Part model, mm, in its own coordinate system. Face numbers are marked on the shaded views. A direction names the side the tool comes from. Coordinates: 2 decimals unless noted, no trailing zeros. Order: outer loops, then holes, each group sorted by start corner. A loop starts at its lowest first (then second) coordinate and runs counter-clockwise, first axis right, second up. Notation, with made-up numbers: M 77,44.5 L 123,44.5 A33 ccw 123,74.5 Z; hole C -10,71.5 d6. An arc over 180 degrees is marked long. Answer in a Markdown table with one row per item. Add a question column.
from build123d import *

# Parameters (mm, degrees)
F0_W     = 6.2
F0_H     = 6.8
F1_DEPTH = 1.5
F2_R     = 1.8
F3_DEPTH = 0.5
F4_R     = 1.5
F5_DEPTH = 1
F6_SIZE  = 0.3


with BuildPart() as f1:
    # F0 (on Top) → F1 (new body)
    with BuildSketch(Plane.XY):
        Rectangle(F0_W, F0_H)
    extrude(amount=F1_DEPTH)

    # F2 (on face) → F3 (cut)
    with BuildSketch(Plane.XY.offset(1.5)):
        Circle(F2_R)
    extrude(amount=-F3_DEPTH, mode=Mode.SUBTRACT)

    # F4 (on face) → F5 (join)
    with BuildSketch(Plane.XY.offset(1)):
        Circle(F4_R)
    extrude(amount=F5_DEPTH)

    # F6
    f6_edges = [f1.edges().sort_by_distance(p)[0] for p in [
        (-3.1, -3.4, 0.75),
        (3.1, -3.4, 0.75),
        (3.1, 3.4, 0.75),
        (-3.1, 3.4, 0.75),
    ]]
    chamfer(f6_edges, length=F6_SIZE)


solid = f1.part
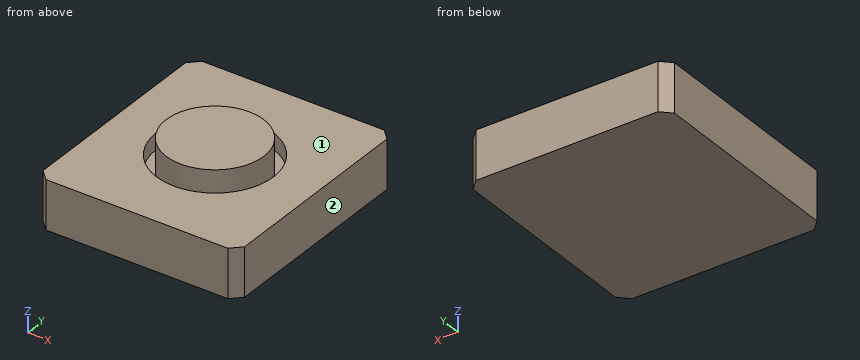
(1) Slice it at C-C (y = 0). List the corners of the cut face in (x, z).
(2) Slice it at D-D (x = 2.25). List the corners of the cut face in (y, z).
(3) Slice it at B-B (x = 0). List the corners of the cut face in (y, z), and give its area (3 significant figures).
(4) Drop flat-ended pins along their axis: P1, Ø2, axis at x = 2, y = -1, coming from the -Z side; P2, Ø2, axis at x = -2, y = 2, coming from the +Z side. Give the stop position or say it passes through.
(5) 3-axis set-ups, long thin cutter, end or side, ignore diameter. For the marked faces 1 and 2: which of +Z, -Z, +X, -X, +Y, -Y reach the whole face in a straight line?
(6) Wall check: line 1 (Y direction, x = 0, z = 1.4); line 2 (Y direction, x = 1, z = 1.35); line 3 (X direction, y = -0.75, z = 1.4). Give the ranges that are in metal, low to high.
(7) Slice it at A-A (z = 1.3). List the corners of the cut face in (x, y).
Computed:
| question | item | result |
|---|---|---|
| 1 | outline | M -3.1,0 L 3.1,0 L 3.1,1.5 L 1.8,1.5 L 1.8,1 L 1.5,1 L 1.5,2 L -1.5,2 L -1.5,1 L -1.8,1 L -1.8,1.5 L -3.1,1.5 Z |
| 2 | outline | M -3.4,0 L 3.4,0 L 3.4,1.5 L -3.4,1.5 Z |
| 3 | outline | M -3.4,0 L 3.4,0 L 3.4,1.5 L 1.8,1.5 L 1.8,1 L 1.5,1 L 1.5,2 L -1.5,2 L -1.5,1 L -1.8,1 L -1.8,1.5 L -3.4,1.5 Z |
| 3 | area | 11.4 mm^2 |
| 4 | P1 | stops at z = 0 |
| 4 | P2 | stops at z = 1.5 |
| 5 | face 1 | +Z |
| 5 | face 2 | +Z, -Z, +X, +Y, -Y |
| 6 | line 1 | y = -3.4 to -1.8, -1.5 to 1.5, 1.8 to 3.4 |
| 6 | line 2 | y = -3.4 to -1.5, -1.12 to 1.12, 1.5 to 3.4 |
| 6 | line 3 | x = -3.1 to -1.64, -1.3 to 1.3, 1.64 to 3.1 |
| 7 | outline | M -3.1,-3.1 L -2.8,-3.4 L 2.8,-3.4 L 3.1,-3.1 L 3.1,3.1 L 2.8,3.4 L -2.8,3.4 L -3.1,3.1 Z; C 0,0 d3; hole C 0,0 d3.6 |
